from build123d import *

# Parameters (mm, degrees)
SKETCH1_R           = 1.6
BOSS_EXTRUDE1_DEPTH = 4
SKETCH2_R           = 3.1
CUT_EXTRUDE1_DEPTH  = 1


with BuildPart() as part:
    # Sketch1 → Boss-Extrude1 (new body)
    with BuildSketch(Plane.XY):
        with BuildLine():
            Line((-12.204375178, -60.110154246), (-12.204375178, -141.110154246))
            ThreePointArc((-12.204375178, -141.110154246), (-10.447015865, -145.352794933), (-6.204375178, -147.110154246))
            Line((-6.204375178, -147.110154246), (117.495624822, -147.110154246))
            ThreePointArc((117.495624822, -147.110154246), (121.738265509, -145.352794933), (123.495624822, -141.110154246))
            Line((123.495624822, -141.110154246), (123.495624822, -60.110154246))
            ThreePointArc((123.495624822, -60.110154246), (121.738265509, -55.867513558), (117.495624822, -54.110154246))
            Line((117.495624822, -54.110154246), (-6.204375178, -54.110154246))
            ThreePointArc((-6.204375178, -54.110154246), (-10.447015865, -55.867513558), (-12.204375178, -60.110154246))
        make_face()
        with Locations((-7.204375178, -58.610154246)):
            Circle(SKETCH1_R, mode=Mode.SUBTRACT)
        with Locations((118.495624822, -58.610154246)):
            Circle(SKETCH1_R, mode=Mode.SUBTRACT)
        with Locations((118.495624822, -142.610154246)):
            Circle(SKETCH1_R, mode=Mode.SUBTRACT)
        with Locations((-7.204375178, -142.610154246)):
            Circle(SKETCH1_R, mode=Mode.SUBTRACT)
    extrude(amount=BOSS_EXTRUDE1_DEPTH)

    # Sketch2 → Cut-Extrude1 (cut)
    with BuildSketch(Plane.XY.offset(4)):
        with Locations((-7.204375178, -58.610154246)):
            Circle(SKETCH2_R)
        with Locations(Location((118.495624822, -58.610154246, 0), (0, 0, 180))):
            Circle(SKETCH2_R)
        with Locations((118.495624822, -142.610154246)):
            Circle(SKETCH2_R)
        with Locations(Location((-7.204375178, -142.610154246, 0), (0, 0, 180))):
            Circle(SKETCH2_R)
    extrude(amount=-CUT_EXTRUDE1_DEPTH, mode=Mode.SUBTRACT)


solid = part.part
Read the model definition and answer for the solid it produces. Units are mm, in the model's axes. A direction names the side the tool comes from. Give positions to 0.01 mm unless a question says otherwise; leave off trailing zeros. Use a Markdown table: item, result.
Q1. A tool of negligible diameter and unlimited length cuts with its end or side. For faces 4 (the face through (-5.77, -61.36, 3.51)), 5 (the face through (-8, -144, 1)), from which of +Z, -Z, +X, -X, +Y, -Y can it reach the whole face along a straight path? Write none if from no direction.
Solved:
| item | result |
|---|---|
| face 4 | +Z |
| face 5 | +Z, -Z |
Q2. Determine the mould class of faces 1 (the face through (55, -100, 4)), 2 (the face through (116.9, -58.5, 1.5)), 3 (the face through (121.78, -55.91, 1.97)) for opening direction Y: pulls with the +Y half, pulls with the -Y half, needs draft (parallel to the pull), parting line crosses it, or undercut.
Solved:
| item | result |
|---|---|
| face 1 | needs draft |
| face 2 | undercut |
| face 3 | pulls with the +Y half |
Q3. This flat-tipped pin is pushed along its axis until it touches: pin 1 (1.9 mm diameter, centred on x = 120, y = -57.5, fed in from +Z). Where does it stop, or does it pass through?
Solved:
| item | result |
|---|---|
| pin 1 | stops at z = 3 |
Q4. Find the intervals of material crossed by line 1 along X through (y, z) = (-59, 1.7); line 2 along X through (y, z) = (-142, 0.3), in increasing order.
Solved:
| item | result |
|---|---|
| line 1 | x = -12.1 to -8.76, -5.65 to 116.94, 120.05 to 123.39 |
| line 2 | x = -12.14 to -8.68, -5.73 to 117.02, 119.97 to 123.43 |
